Model file for the job. Use its own axes, mm. Coordinates: 2 decimals unless noted, no trailing zeros. Loops run counter-clockwise (first coordinate to the right, second up) from the corner with the lowest first, then second, coordinate; pieces in that order, holes last.
from build123d import *

# Parameters (mm, degrees)
F0_R     = 2.921
F1_DEPTH = 1.27


with BuildPart() as f1:
    # F0 (on Top) → F1 (new body, symmetric)
    with BuildSketch(Plane.XY):
        with BuildLine():
            Line((16.008551, -13.481906), (16.008551, 19.728972))
            Line((16.008551, 19.728972), (-3.832283, 19.728972))
            ThreePointArc((-3.832283, 19.728972), (-12.068809, 1.461038), (-31.006849, -5.089415))
            Line((-31.006849, -5.089415), (-31.006849, -13.481906))
            Line((-31.006849, -13.481906), (16.008551, -13.481906))
        make_face()
        with Locations((-26.815849, -9.290906)):
            Circle(F0_R, mode=Mode.SUBTRACT)
        with Locations((0, 15.537972)):
            Circle(F0_R, mode=Mode.SUBTRACT)
    extrude(amount=F1_DEPTH, both=True)


solid = f1.part
Q1. Slice it at A-A (x = 0). List the corners of the cut face in (y, z), and give its area (3 significant figures).
Answers:
outline: (-13.48, -1.27) - (12.62, -1.27) - (12.62, 1.27) - (-13.48, 1.27) - close; (18.46, -1.27) - (19.73, -1.27) - (19.73, 1.27) - (18.46, 1.27) - close
area: 69.5 mm2
Q2. Mould opens along Y. For faces 1 (the cylindrical face through (-0.633, 12.686, -0.018)), 2 (the flat face through (-8, -13.482, 0)), 3 (the cylindrical face through (-29.734, -9.162, -0.018)), 4 (the cylindrical face through (-11.857, 1.657, 0.018)) say: +Y half, -Y half, draft (parallel to the pull), parting line (faces both ways), or undercut.
Answers:
face 1: undercut
face 2: -Y half
face 3: undercut
face 4: +Y half
Q3. Slice it at B-B (y = 13.5). List the corners of the cut face in (x, z).
Answers:
outline: (-4.72, -1.27) - (-2.09, -1.27) - (-2.09, 1.27) - (-4.72, 1.27) - close; (2.09, -1.27) - (16.01, -1.27) - (16.01, 1.27) - (2.09, 1.27) - close
Q4. Flat gauge pin, fed straight in: P1, Ø10, axis at x = -23.5, y = 2.5, coming from the +Z side. Where does the tip first touch, or does it go through?
Answers:
P1: passes through
Q5. Drill centre lines: line 1 (Y direction, x = 0, z = 0.15); line 2 (Y direction, x = -2.5, z = -0.4); line 3 (X direction, y = 16, z = -0.7). Where is each one in solid material? Low to high.
Answers:
line 1: y = -13.48 to 12.62, 18.46 to 19.73
line 2: y = -13.48 to 14.03, 17.05 to 19.73
line 3: x = -4.17 to -2.88, 2.88 to 16.01
Q6. Slice it at C-C (z = 0.35). List the corners of the cut face in (x, y), and give its area (3 significant figures).
Answers:
outline: (-31.01, -13.48) - (16.01, -13.48) - (16.01, 19.73) - (-3.83, 19.73) arc R25.3 cw to (-31.01, -5.09) - close; hole circle Ø5.84 at (-26.82, -9.29); hole circle Ø5.84 at (0, 15.54)
area: 969 mm2
Q7. Slice it at D-D (x = -18). List the corners of the cut face in (y, z).
Answers:
outline: (-13.48, -1.27) - (-2.58, -1.27) - (-2.58, 1.27) - (-13.48, 1.27) - close
